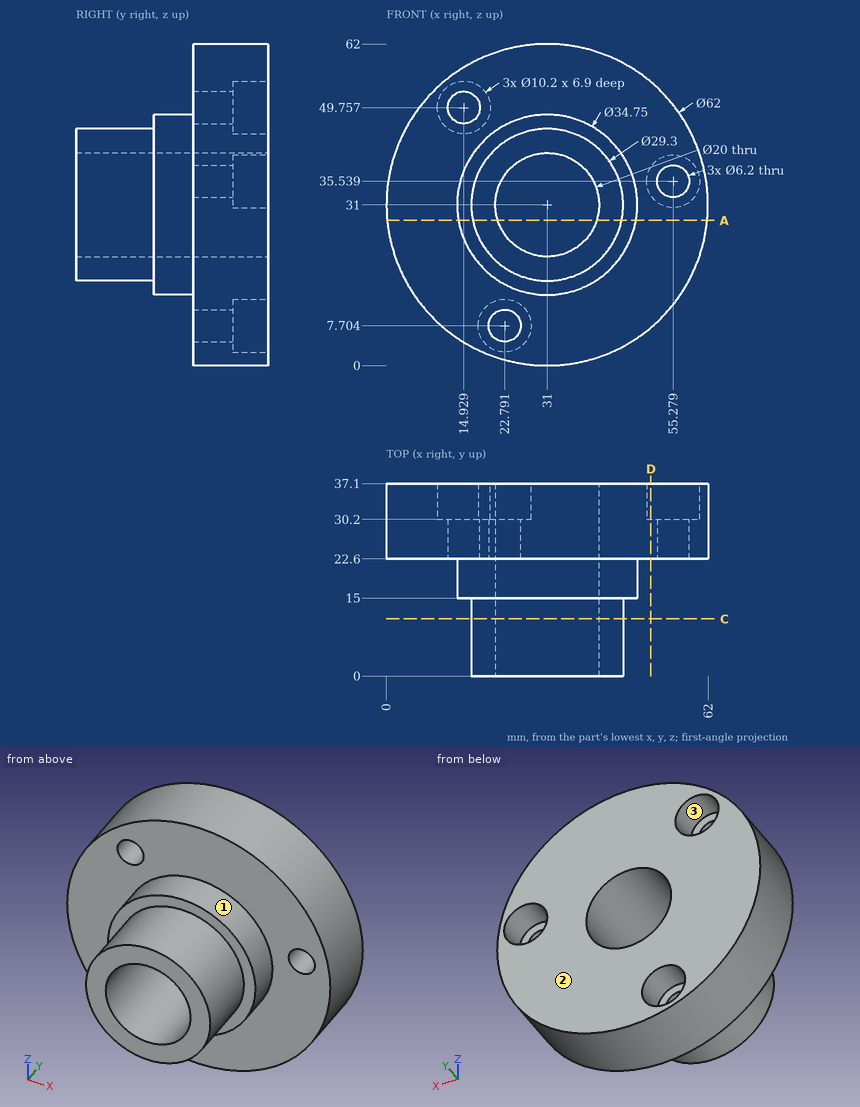
Source: three-view drawing plus pictorial views. Frame: mm from the lowest corner of the part. A direction names the side the tool comes from. Round coordinates to 2 decimals unless told otherwise and drop trailing zeros. Order: outer loops, then holes, each group sorted by start corner. A loop starts at its lowest first (then second) coordinate and runs counter-clockwise, first axis right, second up. Notation, with made-up numbers: (-10.75, -20) -> (29.25, -20) arc R21 ccw to (29.25, 3) -> close; hole circle Ø6 at (66.25, 0.25). An arc over 180 degrees is marked (long way). Use one line per item in the form item = value. Start each with the question number.
1. Line query: probe 1 along Z at (x, y) = (23.5, 27) (1 decimal); probe 2 along Y at (x, z) = (13.5, 39); probe 3 along X at (y, z) = (30.5, 10.5) (1 decimal). Output: solid intervals per line, ascending.
2. Cut plane D-D (x = 51). Return the cut outline in (y, z) (1 decimal).
3. Reachability of the marked faces 1, 2 and 3 from +Z, -Z, +X, -X, +Y, -Y: full face, straight path, thin tool, end or side. Return the list, or none.
4. Cut plane A-A (z = 28). Return the cut outline in (x, y) (1 decimal).
5. Pin query (flat end, axial travel): pin 1 Ø1.5 at (y, z) = (8, 17.5) entering from -X (1 decimal); pin 2 Ø8 at (x, z) = (14.93, 49.76) entering from -Y; pin 3 Ø4 at (y, z) = (29, 32) entering from -X; pin 4 Ø3.5 at (x, z) = (55.28, 35.54) entering from -Y. Return the tip coordinate at first contact, or that it passes through.
6. Cut plane C-C (y = 11). Return the cut outline in (x, z).
Solution:
q1.probe_1 = 0.9 to 4.7, 10.7 to 24.4, 37.6 to 61.1
q1.probe_2 = 22.6 to 37.1
q1.probe_3 = 7.7 to 18.5, 27.1 to 54.3
q2.outline = (22.6, 7.3) -> (37.1, 7.3) -> (37.1, 32.8) -> (30.2, 32.8) -> (30.2, 38.3) -> (37.1, 38.3) -> (37.1, 54.7) -> (22.6, 54.7) -> close
q3.face_1 = -Y
q3.face_2 = +Z, -Z, +X, -X, +Y
q3.face_3 = +Y
q4.outline = (0.1, 22.6) -> (13.9, 22.6) -> (13.9, 15) -> (16.7, 15) -> (16.7, 0) -> (21.5, 0) -> (21.5, 37.1) -> (0.1, 37.1) -> close; (40.5, 0) -> (45.3, 0) -> (45.3, 15) -> (48.1, 15) -> (48.1, 22.6) -> (61.9, 22.6) -> (61.9, 37.1) -> (40.5, 37.1) -> close
q5.pin_1 = 23.8
q5.pin_2 = 22.6
q5.pin_3 = 0
q5.pin_4 = through
q6.outline = circle Ø29.3 at (31, 31); hole circle Ø20 at (31, 31)
